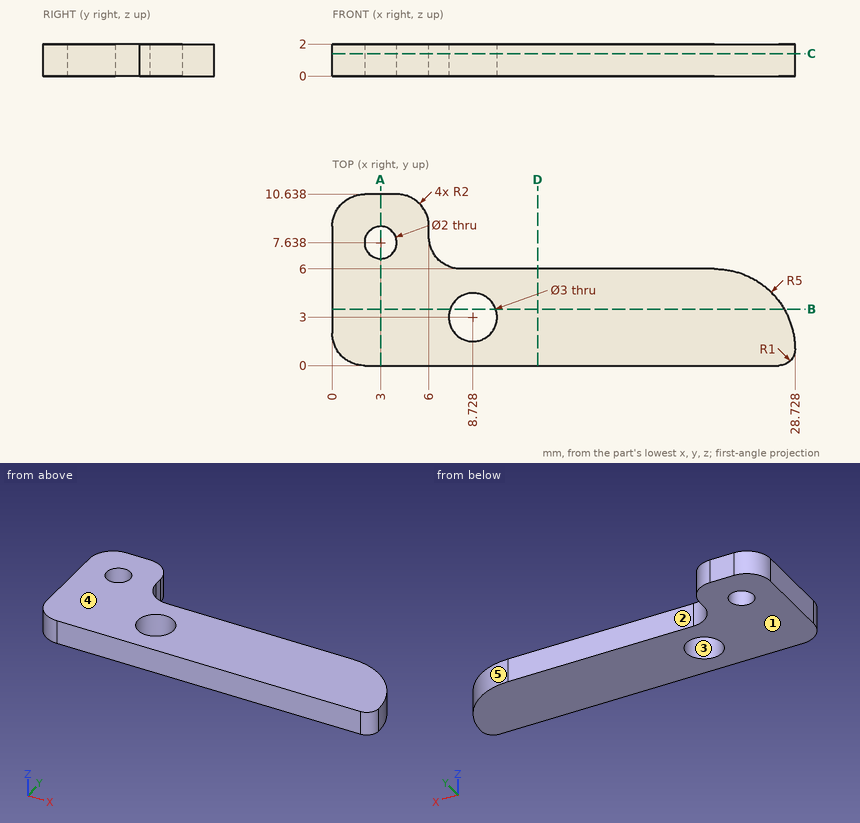
Input: dimensioned drawing with shaded views. Units: mm. Origin: part minimum x, y, z. A direction names the side the tool comes from. Round coordinates to 2 decimals unless told otherwise and drop trailing zeros. Loops run counter-clockwise (first coordinate to the right, second up) from the corner with the lowest first, then second, coordinate; pieces in that order, holes last. Notation, with made-up numbers: (71.5, 12.25) -> (95.5, 12.25) arc R20 cw to (95.5, 24.25) -> close; hole circle Ø6 at (26.5, 42.25). An arc over 180 degrees is marked (long way). Answer as a JSON object with one key per item and string values. Group by question number.
Q1. Section query D-D (x = 12.75). Output: boundary loops of the cut face in (y, z).
Q2. Access query for the marked faces 1 and 2. Directions: +Z, -Z, +X, -X, +Y, -Y. A direction counts if a zero-diameter tool reaches every point of the face in a straight line with its end or side. Return the directions, or none.
Q3. Section query A-A (x = 3). Output: boundary loops of the cut face in (y, z).
Q4. Ray query, line 1 (Y direction, x = 3, z = 0.8); line 2 (X direction, y = 2.75, z = 0.3); line 3 (X direction, y = 1.75, z = 0.85) (1 decimal). Return the intervals inside material, ascending. Write a range as from..to.
Q5. Contact query for flat-ended pins moving along their axis: P1, Ø0.6, axis at x = 19, z = 1, coming from the +Y side; P2, Ø1, axis at y = 2.5, z = 0.5, coming from the -X side; P3, Ø1.8, axis at x = 3, y = 7.64, coming from the -Z side. Output: stop coordinate, or through.
Q6. Mould query, pull axis X, two halves, no side actions, for the marked faces 3, 4 and 5. Classes: pulls with the +X half, pulls with the -X half, needs draft (parallel to the pull), parting line crosses it, or undercut.
Q7. Section query B-B (y = 3.5). Output: boundary loops of the cut face in (x, z).
Q8. Section query C-C (z = 1.4). State how many separate pieces and enclosed holes the cut face has, plus the area to 3 significant figures.
Completed:
{
 "1": {"outline": "(0, 0) -> (6, 0) -> (6, 2) -> (0, 2) -> close"},
 "2": {"face 1": "-Z, +X, -X, +Y, -Y", "face 2": "+Z, -Z, +X, +Y"},
 "3": {"outline": "(0, 0) -> (6.64, 0) -> (6.64, 2) -> (0, 2) -> close; (8.64, 0) -> (10.64, 0) -> (10.64, 2) -> (8.64, 2) -> close"},
 "4": {"line 1": "0..6.64, 8.64..10.64", "line 2": "0..7.25, 10.21..28.41", "line 3": "0..7.9, 9.6..28.7"},
 "5": {"P1": "y = 6", "P2": "x = 0", "P3": "through"},
 "6": {"face 3": "undercut", "face 4": "needs draft", "face 5": "pulls with the +X half"},
 "7": {"outline": "(0, 0) -> (7.31, 0) -> (7.31, 2) -> (0, 2) -> close; (10.14, 0) -> (28.06, 0) -> (28.06, 2) -> (10.14, 2) -> close"},
 "8": {"separate pieces": "1", "enclosed holes": "2", "area": "183 mm²"}
}
